Work out the finished part from the listing and answer in its coordinate system (mm). A direction names the side the tool comes from. Give positions to 0.01 mm unless a question says otherwise; leave off trailing zeros. Write each loop counter-clockwise with the first axis right and the second up, starting at its lowest first coordinate (ties: lowest second). Pieces come first, ordered by that corner, then holes. Notation, with made-up numbers: (47.25, -20.5) -> (101.25, -20.5) arc R13 cw to (101.25, -1.5) -> close; hole circle Ø3 at (32.25, -33.75). An arc over 180 degrees is marked (long way). Write item = value, one per line. Start each with the question number.
from build123d import *

# Parameters (mm, degrees)
F1_DEPTH = 15
F3_DEPTH = 10
F4_R     = 1
F5_R     = 4


with BuildPart() as f1:
    # F0 (on Top) → F1 (new body)
    with BuildSketch(Plane.XY):
        Polygon((100.5, 21), (-100.5, 21), (-100.5, 0), (-62.5, 0), (-56.5, 6), (56.5, 6), (62.5, 0), (100.5, 0), align=None)
    extrude(amount=F1_DEPTH)

    # F2 (on face) → F3 (cut)
    with BuildSketch(Plane.XY.offset(15)):
        Polygon((95.5, 16), (-95.5, 16), (-95.5, 5), (-67.5, 5), (-67.5, 11), (67.5, 11), (67.5, 5), (95.5, 5), align=None)
    extrude(amount=-F3_DEPTH, mode=Mode.SUBTRACT)

    # F4
    f4_edges = [f1.edges().sort_by_distance(p)[0] for p in [
        (67.5, 11, 10),
        (-67.5, 11, 10),
    ]]
    fillet(f4_edges, radius=F4_R)

    # F5
    f5_edges = [f1.edges().sort_by_distance(p)[0] for p in [
        (-62.5, 0, 7.5),
        (-56.5, 6, 7.5),
        (56.5, 6, 7.5),
        (62.5, 0, 7.5),
        (-100.5, 0, 7.5),
        (-100.5, 21, 7.5),
        (100.5, 21, 7.5),
        (100.5, 0, 7.5),
    ]]
    fillet(f5_edges, radius=F5_R)


solid = f1.part
(1) A cutting plane is placed at D-D, the plane y = 8.25. Write down the section's boundary in (x, z).
(2) Find the intervals of material crossed by line 1 along X through (y, z) = (9, 10.75); line 2 along Y through (x, z) = (-49, 8.75); line 3 along Y through (x, z) = (75, 14.25), in increasing order.
(3) A cutting plane is placed at B-B, the plane x = 70. Write down the section's boundary in (y, z).
(4) This flat-tipped pin is pushed along its axis until it touches: pin 1 (3 mm diameter, centred on x = 15.5, z = 4.5, fed in from -Y). Where does it stop, or does it pass through?
(5) A cutting plane is placed at C-C, the plane z = 2.5. Write down the section's boundary in (x, y).
(6) Determine the mould class of faces 1 (the flat face through (-59.5, 3, 7.4)), 2 (the cylindrical face through (99.359, 1.203, 7.605)), 3 (the cylindrical face through (-99.297, 19.859, 7.605)) for opening direction X: pulls with the +X half, pulls with the -X half, needs draft (parallel to the pull), parting line crosses it, or undercut.
(7) A cutting plane is placed at A-A, the plane z = 10.5. Write down the section's boundary in (x, y), then the cut area to 3 significant figures.
(8) For faces 4 (the flat face through (-82, 5, 10)), 5 (the flat face through (-1, 6, 7)), 6 (the cylindrical face through (99.297, 19.859, 7.605)), determine the directions among +Z, -Z, +X, -X, +Y, -Y from which every point of the face is accessible in a straight line to the end or side of a thin tool.
Results list:
q1.outline = (-100.5, 0) -> (100.5, 0) -> (100.5, 15) -> (95.5, 15) -> (95.5, 5) -> (67.5, 5) -> (67.5, 15) -> (-67.5, 15) -> (-67.5, 5) -> (-95.5, 5) -> (-95.5, 15) -> (-100.5, 15) -> close
q2.line_1 = -100.5 to -95.5, -67.5 to 67.5, 95.5 to 100.5
q2.line_2 = 6 to 11, 16 to 21
q2.line_3 = 0 to 5, 16 to 21
q3.outline = (0, 0) -> (21, 0) -> (21, 15) -> (16, 15) -> (16, 5) -> (5, 5) -> (5, 15) -> (0, 15) -> close
q4.pin_1 = 6
q5.outline = (-100.5, 4) arc R4 ccw to (-96.5, 0) -> (-64.16, 0) arc R4 ccw to (-61.33, 1.17) -> (-57.67, 4.83) arc R4 cw to (-54.84, 6) -> (54.84, 6) arc R4 cw to (57.67, 4.83) -> (61.33, 1.17) arc R4 ccw to (64.16, 0) -> (96.5, 0) arc R4 ccw to (100.5, 4) -> (100.5, 17) arc R4 ccw to (96.5, 21) -> (-96.5, 21) arc R4 ccw to (-100.5, 17) -> close
q6.face_1 = undercut
q6.face_2 = pulls with the +X half
q6.face_3 = pulls with the -X half
q7.outline = (-100.5, 4) arc R4 ccw to (-96.5, 0) -> (-64.16, 0) arc R4 ccw to (-61.33, 1.17) -> (-57.67, 4.83) arc R4 cw to (-54.84, 6) -> (54.84, 6) arc R4 cw to (57.67, 4.83) -> (61.33, 1.17) arc R4 ccw to (64.16, 0) -> (96.5, 0) arc R4 ccw to (100.5, 4) -> (100.5, 17) arc R4 ccw to (96.5, 21) -> (-96.5, 21) arc R4 ccw to (-100.5, 17) -> close; hole (-95.5, 5) -> (-67.5, 5) -> (-67.5, 10) arc R1 cw to (-66.5, 11) -> (66.5, 11) arc R1 cw to (67.5, 10) -> (67.5, 5) -> (95.5, 5) -> (95.5, 16) -> (-95.5, 16) -> close
q7.area = 2,200 mm²
q8.face_4 = +Z
q8.face_5 = +Z, -Z, -Y
q8.face_6 = +Z, -Z, +X, +Y
